from build123d import *

# Parameters (mm, degrees)
BOSS_EXTRUDE1_DEPTH = 100
SKETCH2_R           = 1.5
CUT_EXTRUDE1_DEPTH  = 20


with BuildPart() as part:
    # Sketch1 → Boss-Extrude1 (new body)
    with BuildSketch(Plane.XY):
        Polygon((-10, 2.6), (-7.7, 2.6), (-7.7, 5), (-6.767766953, 5), (-4.4, 2.632233047), (-4.4, -2.632233047), (-6.767766953, -5), (-7.7, -5), (-7.7, -2.6), (-10, -2.6), align=None)
    extrude(amount=BOSS_EXTRUDE1_DEPTH)

    # Sketch2 → Cut-Extrude1 (cut)
    with BuildSketch(Plane.ZY.offset(10)):
        with Locations((83.3, 0)):
            Circle(SKETCH2_R)
        with Locations((66.7, 0)):
            Circle(SKETCH2_R)
        with Locations(Location((16.7, 0, 0), (0, 0, 270))):
            Circle(SKETCH2_R)
        with Locations(Location((33.3, 0, 0), (0, 0, 270))):
            Circle(SKETCH2_R)
    extrude(amount=-CUT_EXTRUDE1_DEPTH, mode=Mode.SUBTRACT)


solid = part.part
CAD build for the part. Positions are in the model's coordinates, mm. A direction names the side the tool comes from. Round coordinates to 2 decimals unless told otherwise and drop trailing zeros. Order: outer loops, then holes, each group sorted by start corner. A loop starts at its lowest first (then second) coordinate and runs counter-clockwise, first axis right, second up. Notation, with made-up numbers: (81, 29.25) - (134, 29.25) arc R35 ccw to (134, 68.25) - close; hole circle Ø4 at (46.5, 23.5). An arc over 180 degrees is marked (long way). Return JSON: item names as keys, results as strings.
(1) Cut at A-A (z = 33.3). Give the cut face in (x, y).
Answer key:
{"outline": "(-10, -2.6) - (-7.7, -2.6) - (-7.7, -5) - (-6.77, -5) - (-4.4, -2.63) - (-4.4, -1.5) - (-10, -1.5) - close; (-10, 1.5) - (-4.4, 1.5) - (-4.4, 2.63) - (-6.77, 5) - (-7.7, 5) - (-7.7, 2.6) - (-10, 2.6) - close"}
(2) Cut at B-B (y = 0). Give the cut face in (x, z), then the cut area to 3 significant figures.
Answer key:
{"outline": "(-10, 0) - (-4.4, 0) - (-4.4, 15.2) - (-10, 15.2) - close; (-10, 18.2) - (-4.4, 18.2) - (-4.4, 31.8) - (-10, 31.8) - close; (-10, 34.8) - (-4.4, 34.8) - (-4.4, 65.2) - (-10, 65.2) - close; (-10, 68.2) - (-4.4, 68.2) - (-4.4, 81.8) - (-10, 81.8) - close; (-10, 84.8) - (-4.4, 84.8) - (-4.4, 100) - (-10, 100) - close", "area": "493 mm^2"}
(3) Pull direction Z, two halves, no side cores. Call faces 4 (the face through (-7, 0, 0)), 5 (the face through (-7.239, 1.265, 84.106)), 6 (the face through (-4.4, 0, 49)): +Z half, -Z half, draft (parallel to the pull), parting line (faces both ways), or undercut.
Answer key:
{"face 4": "-Z half", "face 5": "undercut", "face 6": "draft"}
(4) Tool access for faces 1 (the face through (-7, 0, 100)), 2 (the face through (-9, 2.6, 49)), 3 (the face through (-9, -2.6, 49)): list every direction of +Z, -Z, +X, -X, +Y, -Y with a clear straight run to the whole face (end or side of a thin tool).
Answer key:
{"face 1": "+Z, +X, -X, +Y, -Y", "face 2": "+Z, -Z, -X, +Y", "face 3": "+Z, -Z, -X, -Y"}
(5) Cut at C-C (x = -5.55). Give the cut face in (y, z), then the cut area to 3 significant figures.
Answer key:
{"outline": "(-3.78, 0) - (3.78, 0) - (3.78, 100) - (-3.78, 100) - close; hole circle Ø3 at (0, 16.7); hole circle Ø3 at (0, 33.3); hole circle Ø3 at (0, 66.7); hole circle Ø3 at (0, 83.3)", "area": "728 mm^2"}
(6) Pin check, flat tips, straight feed: pin 1 Ø4 at (y, z) = (0, 16.7) entering from -X; pin 2 Ø1.2 at (x, z) = (-8.5, 45.5) entering from +Y; pin 3 Ø1.2 at (y, z) = (-4, 36.5) entering from -X. Stop position of each tip, or through.
Answer key:
{"pin 1": "stops at x = -10", "pin 2": "stops at y = 2.6", "pin 3": "stops at x = -7.7"}
(7) Wall check: probe 1 along Y at (x, z) = (-8.6, 66.7); probe 2 along Z at (x, y) = (-5.45, 0.25); probe 3 along Y at (x, z) = (-8.4, 55.5). Give the ranges that are in metal, low to high. Write a range as from..to.
Answer key:
{"probe 1": "y = -2.6..-1.5, 1.5..2.6", "probe 2": "z = 0..15.22, 18.18..31.82, 34.78..65.22, 68.18..81.82, 84.78..100", "probe 3": "y = -2.6..2.6"}
